Verification items for the finished model (mm, model axes). Coordinates: 2 decimals unless noted, no trailing zeros. Write each loop counter-clockwise with the first axis right and the second up, starting at its lowest first coordinate (ties: lowest second). Pieces come first, ordered by that corner, then holes. Notation, with made-up numbers: M 5.25,9.25 L 57.25,9.25 A21 ccw 57.25,24.25 Z; hole C 71.25,-13 d3. An arc over 180 degrees is marked long. Answer in a Markdown table with one row per item.
from build123d import *

# Parameters (mm, degrees)
F1_DEPTH = 45.72


with BuildPart() as f1:
    # F0 (on Front) → F1 (new body)
    with BuildSketch(Plane.XZ):
        with BuildLine():
            Line((0, 114.3), (0, 0))
            Line((0, 0), (62.23, 0))
            Line((62.23, 0), (62.23, 114.3))
            Line((62.23, 114.3), (45.085, 114.3))
            ThreePointArc((45.085, 114.3), (31.115, 100.33), (17.145, 114.3))
            Line((17.145, 114.3), (0, 114.3))
        make_face()
    extrude(amount=-F1_DEPTH)


solid = f1.part
1) Thickness scan on L1, parallel to Z at x = 30.5, y = 7; L2, parallel to Z at x = 20.5, y = 8. Record the ranges inside material, lowest first. Write a range as [from, to].
Response values:
| item | result |
|---|---|
| L1 | z = [0, 100.34] |
| L2 | z = [0, 105.22] |
2) Sectioned sample at C-C (x = 41.5). Record the cut outline in (y, z), then the cut area to 3 significant figures.
Response values:
| item | result |
|---|---|
| outline | M 0,0 L 45.72,0 L 45.72,104.96 L 0,104.96 Z |
| area | 4,800 mm² |
3) Release check for a two-part mould opening along X. For faces 1 (the face through (31, 23, 0)), 2 (the face through (62.23, 23, 56)), 3 (the face through (31.422, 22.54, 100.333)) record: +X half, -X half, draft (parallel to the pull), parting line (faces both ways), or undercut.
Response values:
| item | result |
|---|---|
| face 1 | draft |
| face 2 | +X half |
| face 3 | undercut |
4) Sectioned sample at B-B (x = 22). Record the cut outline in (y, z), then the cut area to 3 significant figures.
Response values:
| item | result |
|---|---|
| outline | M 0,0 L 45.72,0 L 45.72,103.71 L 0,103.71 Z |
| area | 4,740 mm² |
5) Sectioned sample at A-A (y = 6.5). Record the cut outline in (x, z) (3 decimals).
Response values:
| item | result |
|---|---|
| outline | M 0,0 L 62.23,0 L 62.23,114.3 L 45.085,114.3 A13.97 cw 17.145,114.3 L 0,114.3 Z |
